Could you check a few things on this model? Use its own coordinates, in mm. A direction names the side the tool comes from. Give positions to 0.01 mm unless a question says otherwise; leave off trailing zeros. Order: outer loops, then holes, each group sorted by start corner. A loop starts at its lowest first (then second) coordinate and runs counter-clockwise, first axis right, second up. Notation, with made-up numbers: (68.25, 59.5) - (79.25, 59.5) arc R20 ccw to (79.25, 81.5) - close; hole circle Ø6 at (-20.75, -12). An arc over 180 degrees is marked (long way). One line per question, with ' | ' between items. Start each with the question number.
1. I need wall thicknesses on probe 1 along X at (y, z) = (-4, 0); probe 2 along Z at (x, y) = (89, -2); probe 3 along Y at (x, z) = (12, 8.5). Which ranges of each line are inside material? Lowest first, please. Write a range as from..to.
2. If we mould it in two halves opening along Z, with no side actions, what happens to faces 6 (the flat face through (-1, 0, -5)), 7 (the flat face through (-9.3, 9, -5.2)), 8 (the cylindrical face through (71.412, 0.126, 10.227))? For each: released by +Z, released by -Z, zero draft, split by the parting line, or undercut.
3. Imagine slicing it at A-A (x = 58). Please give me the cut outline in (y, z).
4. Imagine slicing it at C-C (z = 0). Please give me the cut outline in (x, y), and give its area (3 significant figures).
5. Which directions (+Z, -Z, +X, -X, +Y, -Y) give clear straight access to the entire face, cutting with the end or side of a thin tool? Please do faces 1 (the flat face through (-6, 0, 9)), 2 (the flat face through (-94, -14, -6)), 3 (the cylindrical face through (-79.44, 0.13, -9.49)), 4 (the flat face through (1, 0, 5)), 5 (the cylindrical face through (106.084, 0.294, 3.794)).
6. Imagine slicing it at B-B (y = -0.5). Please give me the cut outline in (x, z), and give its area (3 significant figures).
7. For P1, Ø14.5, axis at x = 8.5, y = -1, coming from the +Z side; P2, Ø4, axis at x = 20, y = 10, coming from the -Z side; P3, Ø12, axis at y = 14.5, z = -9, coming from the +X side, each with a flat end and sliding along its axis, tell me the tip position at first contact or that it passes through.
8. Imagine slicing it at D-D (y = -17.5). Please give me the cut outline in (x, z), and give its area (3 significant figures).
```python
from build123d import *

# Parameters (mm, degrees)
SKETCH1_R           = 12
SKETCH1_R_2         = 7.5
BOSS_EXTRUDE1_DEPTH = 14
SKETCH1_6_R         = 17.5
SKETCH1_6_R_2       = 12
BOSS_EXTRUDE2_DEPTH = 21
BOSS_EXTRUDE3_DEPTH = 9
CUT_EXTRUDE1_REACH  = 114.02


with BuildPart() as part:
    # Sketch1 → Boss-Extrude1 (new, symmetric)
    with BuildSketch(Plane(origin=(0, 0, 0), x_dir=(1, 0, 0), z_dir=(0, 1, 0))):
        with Locations(Location((-89, 0, 0), (0, 0, 270))):
            Circle(SKETCH1_R)
        with Locations(Location((-89, 0, 0), (0, 0, 270))):
            Circle(SKETCH1_R_2, mode=Mode.SUBTRACT)
    extrude(amount=BOSS_EXTRUDE1_DEPTH, both=True)



with BuildPart() as body_2:
    # Sketch1_6 → Boss-Extrude2 (new, symmetric)
    with BuildSketch(Plane(origin=(0, 0, 0), x_dir=(1, 0, 0), z_dir=(0, 1, 0))):
        with Locations(Location((89, 0, 0), (0, 0, 90))):
            Circle(SKETCH1_6_R)
        with Locations(Location((89, 0, 0), (0, 0, 90))):
            Circle(SKETCH1_6_R_2, mode=Mode.SUBTRACT)
    extrude(amount=BOSS_EXTRUDE2_DEPTH, both=True)


with BuildPart() as part_1:
    add(part.part)

    add(body_2.part)  # Boss-Extrude3 merges body 2
    # Sketch1_7 → Boss-Extrude3 (add, symmetric)
    with BuildSketch(Plane(origin=(0, 0, 0), x_dir=(1, 0, 0), z_dir=(0, 1, 0))):
        with BuildLine():
            ThreePointArc((-84.204168477, 11), (-78.96132533, 6.574573055), (-77, 0))
            Line((-77, 0), (71.5, 0))
            ThreePointArc((71.5, 0), (73.316384657, 7.76364668), (78.388481117, 13.915662651))
            ThreePointArc((78.388481117, 13.915662651), (71.515902373, 10.26210106), (63.835540936, 9))
            Line((63.835540936, 9), (-74.61250543, 9))
            ThreePointArc((-74.61250543, 9), (-79.511484916, 9.505319751), (-84.204168477, 11))
        make_face()
        with BuildLine():
            Line((71.5, 0), (-77, 0))
            ThreePointArc((-77, 0), (-78.96132533, -6.574573055), (-84.204168477, -11))
            ThreePointArc((-84.204168477, -11), (-79.511484916, -9.505319751), (-74.61250543, -9))
            Line((-74.61250543, -9), (63.835540936, -9))
            ThreePointArc((63.835540936, -9), (71.515902373, -10.26210106), (78.388481117, -13.915662651))
            ThreePointArc((78.388481117, -13.915662651), (73.316384657, -7.76364668), (71.5, 0))
        make_face()
    extrude(amount=BOSS_EXTRUDE3_DEPTH, both=True)

    # Sketch2 → Cut-Extrude1 (cut, up to next)
    with BuildSketch(Plane(origin=(0, 9, 0), x_dir=(1, 0, 0), z_dir=(0, 1, 0)), mode=Mode.PRIVATE) as cut_extrude1_sk1:
        with BuildLine():
            Line((-65, 5), (65, 5))
            ThreePointArc((65, 5), (70, 0), (65, -5))
            Line((65, -5), (-65, -5))
            ThreePointArc((-65, -5), (-70, 0), (-65, 5))
        make_face()
    cut_extrude1_tool1 = extrude(cut_extrude1_sk1.sketch, amount=-CUT_EXTRUDE1_REACH, mode=Mode.PRIVATE) & part_1.part
    add(cut_extrude1_tool1.solids().sort_by_distance((0, 9, 0))[0], mode=Mode.SUBTRACT)


solid = part_1.part
```
Results found:
1) probe 1: x = -101..-96.5, -81.5..-70, 70..77, 101..106.5 | probe 2: z = -17.5..-12, 12..17.5 | probe 3: y = -9..9
2) face 6: undercut | face 7: zero draft | face 8: released by +Z
3) outline: (-9, -9) - (9, -9) - (9, -5) - (-9, -5) - close; (-9, 5) - (9, 5) - (9, 9) - (-9, 9) - close
4) outline: (-101, -14) - (-96.5, -14) - (-96.5, 14) - (-101, 14) - close; (-81.5, -14) - (-77, -14) - (-77, -9) - (-70, -9) - (-70, 9) - (-77, 9) - (-77, 14) - (-81.5, 14) - close; (70, -9) - (71.5, -9) - (71.5, -21) - (77, -21) - (77, 21) - (71.5, 21) - (71.5, 9) - (70, 9) - close; (101, -21) - (106.5, -21) - (106.5, 21) - (101, 21) - close | area: 867 mm2
5) face 1: +Z, +Y, -Y | face 2: +Z, -Z, -X, -Y | face 3: -Z, +Y, -Y | face 4: +Y, -Y | face 5: none
6) outline: (-84.2, -11) arc R24 cw to (-74.61, -9) - (63.84, -9) arc R24 cw to (78.39, -13.92) arc R17.5 ccw (long way) to (78.39, 13.92) arc R24 cw to (63.84, 9) - (-74.61, 9) arc R24 cw to (-84.2, 11) arc R12 ccw (long way) to start; hole circle Ø15 at (-89, 0); hole (-65, -5) - (65, -5) arc R5 ccw to (65, 5) - (-65, 5) arc R5 ccw to start; hole circle Ø24 at (89, 0) | area: 2,140 mm2
7) P1: stops at z = 9 | P2: stops at z = -9 | P3: stops at x = 106.24
8) outline: circle Ø35 at (89, 0); hole circle Ø24 at (89, 0) | area: 510 mm2
